Design review of the part built by this model. Coordinates are the model's own, in mm. A direction names the side the tool comes from. Coordinates: 2 decimals unless noted, no trailing zeros. Loops run counter-clockwise (first coordinate to the right, second up) from the corner with the lowest first, then second, coordinate; pieces in that order, holes last.
from build123d import *

# Parameters (mm, degrees)
BOSS_EXTRUDE1_DEPTH = 200
FILLET1_R           = 50
FILLET2_R           = 10
FILLET3_R           = 40
FILLET4_R           = 5
FILLET5_R           = 5
FILLET6_R           = 1
FILLET7_R           = 1
FILLET8_R           = 1
FILLET10_R          = 10
SHELL3_START        = 2
SHELL3_DEPTH        = 196
FILLET14_R          = 1
FILLET15_R          = 1
SKETCH5_W           = 165
SKETCH5_H           = 105
CUT_EXTRUDE1_DEPTH  = 20
SKETCH6_W           = 10
SKETCH6_H           = 3
CUT_EXTRUDE4_DEPTH  = 23
SKETCH8_R           = 7
CUT_EXTRUDE6_DEPTH  = 10
SKETCH9_R           = 10
SKETCH9_R_2         = 7.5
CUT_EXTRUDE7_DEPTH  = 3
SKETCH10_W          = 108
SKETCH10_H          = 2.810580917
SKETCH10_H_2        = 2.810580918
CUT_EXTRUDE8_DEPTH  = 3


# Read off the part's stored shape, not the designer's step: Shell3
with BuildPart() as part:
    # Sketch3 → Boss-Extrude1 (new body)
    with BuildSketch(Plane(origin=(0, 0, 0), x_dir=(0, 0, -1), z_dir=(1, 0, 0))):
        Polygon((-61.287916817, 93.76136528), (-140.28529736, -56.769076383), (39.71470264, -56.769076383), (39.71470264, -26.769076383), (0, -20.093366582), (0, 64.906633418), (22.555153974, 64.906633418), (22.555153974, 74.906633418), (4.646904738, 74.906633418), (4.646904738, 93.76136528), align=None)
    extrude(amount=BOSS_EXTRUDE1_DEPTH)

    # Fillet1
    fillet1_edges = [part.edges().sort_by_distance(p)[0] for p in [
        (100, 93.76136528, 61.287916817),
    ]]
    fillet(fillet1_edges, radius=FILLET1_R)

    # Fillet2
    fillet2_edges = [part.edges().sort_by_distance(p)[0] for p in [
        (100, -56.769076383, 140.28529736),
    ]]
    fillet(fillet2_edges, radius=FILLET2_R)

    # Fillet3
    fillet3_edges = [part.edges().sort_by_distance(p)[0] for p in [
        (100, -20.093366582, 0),
    ]]
    fillet(fillet3_edges, radius=FILLET3_R)

    # Fillet4
    fillet4_edges = [part.edges().sort_by_distance(p)[0] for p in [
        (100, -26.769076383, -39.71470264),
    ]]
    fillet(fillet4_edges, radius=FILLET4_R)

    # Fillet5
    fillet5_edges = [part.edges().sort_by_distance(p)[0] for p in [
        (100, 74.906633418, -4.646904738),
    ]]
    fillet(fillet5_edges, radius=FILLET5_R)

    # Fillet6
    fillet6_edges = [part.edges().sort_by_distance(p)[0] for p in [
        (100, 93.76136528, -4.646904738),
    ]]
    fillet(fillet6_edges, radius=FILLET6_R)

    # Fillet7
    fillet7_edges = [part.edges().sort_by_distance(p)[0] for p in [
        (100, 74.906633418, -22.555153974),
    ]]
    fillet(fillet7_edges, radius=FILLET7_R)

    # Fillet8
    fillet8_edges = [part.edges().sort_by_distance(p)[0] for p in [
        (100, 64.906633418, -22.555153974),
    ]]
    fillet(fillet8_edges, radius=FILLET8_R)

    # Fillet10
    fillet10_edges = [part.edges().sort_by_distance(p)[0] for p in [
        (100, 64.906633418, 0),
    ]]
    fillet(fillet10_edges, radius=FILLET10_R)

    # Shell3 outline → Shell3 (cut)
    with BuildSketch(Plane.YZ.offset(SHELL3_START)):
        with BuildLine():
            Line((-27.674806697, -33.037823142), (-25.702476507, -33.369355374))
            ThreePointArc((-25.702476507, -33.369355374), (-12.089709184, -9.461288624), (13.744127299, 0))
            Line((13.744127299, 0), (54.906633418, 0))
            Line((54.906633418, 0), (54.906633418, 2))
            ThreePointArc((54.906633418, 2), (63.391914792, -1.514718626), (66.906633418, -10))
            Line((66.906633418, -10), (66.906633418, -20.555153974))
            Line((66.906633418, -20.555153974), (72.906633418, -20.555153974))
            Line((72.906633418, -20.555153974), (72.906633418, -9.646904738))
            ThreePointArc((72.906633418, -9.646904738), (74.956885949, -4.697157269), (79.906633418, -2.646904738))
            Line((79.906633418, -2.646904738), (91.76136528, -2.646904738))
            Line((91.76136528, -2.646904738), (91.76136528, 31.060602511))
            ThreePointArc((91.76136528, 31.060602511), (84.838407844, 55.893576038), (66.066508022, 73.563315451))
            Line((66.066508022, 73.563315451), (-43.051552593, 130.82775222))
            ThreePointArc((-43.051552593, 130.82775222), (-50.907905305, 130.590140491), (-54.769076383, 123.74396673))
            Line((-54.769076383, 123.74396673), (-54.769076383, -37.71470264))
            Line((-54.769076383, -37.71470264), (-30.998763119, -37.71470264))
            ThreePointArc((-30.998763119, -37.71470264), (-29.061225382, -37.005105993), (-28.040267833, -35.212000987))
            Line((-28.040267833, -35.212000987), (-27.674806697, -33.037823142))
        make_face()
    extrude(amount=SHELL3_DEPTH, mode=Mode.SUBTRACT)

    # Fillet14
    fillet14_edges = [part.edges().sort_by_distance(p)[0] for p in [
        (200, -43.883919751, -39.71470264),
        (200, 12.436858662, 103.966480208),
        (200, 86.549951284, 56.928283268),
        (200, -56.769076383, 42.014632045),
        (200, -51.942612535, 132.301683931),
        (200, 34.325380359, 0),
        (200, -12.089709184, -9.461288624),
        (200, -25.885207075, -34.456444296),
        (200, -27.769533558, -38.532041562),
        (200, 86.333999349, -4.646904738),
        (200, 76.371099512, -6.111370832),
        (200, 93.76136528, 13.706848886),
        (200, 93.468472061, -4.354011519),
        (200, 74.906633418, -15.601029356),
        (200, 74.613740199, -22.262260756),
        (200, 69.906633418, -22.555153974),
        (200, 65.199526636, -22.262260756),
        (200, 64.906633418, -15.777576987),
        (200, 61.97770123, -2.928932188),
    ]]
    fillet(fillet14_edges, radius=FILLET14_R)

    # Fillet15
    fillet15_edges = [part.edges().sort_by_distance(p)[0] for p in [
        (0, -43.883919751, -39.71470264),
        (0, 12.436858662, 103.966480208),
        (0, 86.549951284, 56.928283268),
        (0, -56.769076383, 42.014632045),
        (0, -51.942612535, 132.301683931),
        (0, 34.325380359, 0),
        (0, -12.089709184, -9.461288624),
        (0, -25.885207075, -34.456444296),
        (0, -27.769533558, -38.532041562),
        (0, 86.333999349, -4.646904738),
        (0, 76.371099512, -6.111370832),
        (0, 93.76136528, 13.706848886),
        (0, 93.468472061, -4.354011519),
        (0, 74.906633418, -15.601029356),
        (0, 74.613740199, -22.262260756),
        (0, 69.906633418, -22.555153974),
        (0, 65.199526636, -22.262260756),
        (0, 64.906633418, -15.777576987),
        (0, 61.97770123, -2.928932188),
    ]]
    fillet(fillet15_edges, radius=FILLET15_R)

    # Sketch5 → Cut-Extrude1 (cut)
    with BuildSketch(Plane(origin=(0, 45.46476773, 86.633651895), x_dir=(1, 0, 0), z_dir=(0, 0.4646904737791423, 0.8854731862563182))):
        with Locations((100, -28.184050547)):
            Rectangle(SKETCH5_W, SKETCH5_H)
    extrude(amount=-CUT_EXTRUDE1_DEPTH, mode=Mode.SUBTRACT)

    # Sketch6 → Cut-Extrude4 (cut)
    with BuildSketch(Plane(origin=(0, 74.906633418, 0), x_dir=(1, 0, 0), z_dir=(0, 1, 0))):
        with Locations((179, 17.055153974)):
            Rectangle(SKETCH6_W, SKETCH6_H)
        with Locations((139, 17.055153974)):
            Rectangle(SKETCH6_W, SKETCH6_H)
        with Locations((99, 17.055153974)):
            Rectangle(SKETCH6_W, SKETCH6_H)
        with Locations((59, 17.055153974)):
            Rectangle(SKETCH6_W, SKETCH6_H)
        with Locations((19, 17.021146207)):
            Rectangle(SKETCH6_W, SKETCH6_H)
    extrude(amount=-CUT_EXTRUDE4_DEPTH, mode=Mode.SUBTRACT)

    # Sketch8 → Cut-Extrude6 (cut)
    with BuildSketch(Plane(origin=(0, 45.46476773, 86.633651895), x_dir=(1, 0, 0), z_dir=(0, 0.4646904737791423, 0.8854731862563182))):
        with Locations(Location((31, -90.684050547, 0), (0, 0, 270))):
            Circle(SKETCH8_R)
        with Locations(Location((169, -90.684050547, 0), (0, 0, 270))):
            Circle(SKETCH8_R)
    extrude(amount=-CUT_EXTRUDE6_DEPTH, mode=Mode.SUBTRACT)

    # Sketch9 → Cut-Extrude7 (cut)
    with BuildSketch(Plane(origin=(0, 0, -39.71470264), x_dir=(-1, 0, 0), z_dir=(0, 0, -1))):
        with Locations(Location((-179, -44.269076383, 0), (0, 0, 90))):
            Circle(SKETCH9_R)
        with Locations(Location((-149, -44.039846818, 0), (0, 0, 90))):
            Circle(SKETCH9_R)
        with Locations(Location((-119, -44.039846818, 0), (0, 0, 90))):
            Circle(SKETCH9_R)
        with Locations(Location((-89, -43.960489904, 0), (0, 0, 90))):
            Circle(SKETCH9_R)
        with Locations(Location((-59, -43.960489904, 0), (0, 0, 90))):
            Circle(SKETCH9_R)
        with Locations(Location((-21, -41.769076383, 0), (0, 0, 90))):
            Circle(SKETCH9_R_2)
    extrude(amount=-CUT_EXTRUDE7_DEPTH, mode=Mode.SUBTRACT)

    # Sketch10 → Cut-Extrude8 (cut)
    with BuildSketch(Plane(origin=(0, 45.46476773, 86.633651895), x_dir=(1, 0, 0), z_dir=(0, 0.46469047377914224, 0.8854731862563181))):
        with Locations((100, -87.49160573)):
            Rectangle(SKETCH10_W, SKETCH10_H)
        with Locations((100, -91.302186647)):
            Rectangle(SKETCH10_W, SKETCH10_H_2)
        with Locations((100, -95.112767565)):
            Rectangle(SKETCH10_W, SKETCH10_H_2)
    extrude(amount=-CUT_EXTRUDE8_DEPTH, mode=Mode.SUBTRACT)


solid = part.part
Q1. Take a section at B-B, the plane x = 59. Give the number of separate pieces and of enclosed holes in the cut face, then the cut area to 3 significant figures.
Q2. Take a section at A-A, the plane z = 15. Write out the cut boundary in (x, y), then the cut area to 3 significant figures.
Q3. Clearance check with flat-ended pins moving along their axes: pin 1 Ø1 at (x, y) = (60, 73.5) entering from +Z; pin 2 Ø9 at (x, y) = (95, 70.5) entering from -Z; pin 3 Ø0.5 at (x, y) = (198.5, 27.5) entering from -Z. State where each tip first meets the part, or that it passes through.
Q4. Machinability: for faces 1 (the cylindrical face through (101.39, 62.06, -3.01)), 2 (the flat face through (99, 91.761, 14)), 3 (the cylindrical face through (127.43, -38.66, -38.73)), which of the approach directions +Z, -Z, +X, -X, +Y, -Y give a long, thin tool a straight path to every point of the face, cutting with its end or side? Answer none if there is none.
Q5. The part is to be moulded in two halves that separate along Y. For faces 4 (the flat face through (106.87, -27.72, 125.04)), 5 (the cylindrical face through (37.94, -34.48, 127.48)), 6 (the flat face through (99, -47, -39.715)), 7 (the cylindrical face through (52.92, -51.9, -38.73)), say which applies: pulls with the +Y half, pulls with the -Y half, needs draft (parallel to the pull), parting line crosses it, or undercut.
Q6. For line 1 (Y direction, x = 117, z = -20); line 2 (Y direction, x = 86, z = 8); line 3 (X direction, y = 20.5, z = 18.5), list the stretches that pass through material, from the lowest coordinate up.
Entries:
1. separate pieces: 8
1. enclosed holes: 0
1. area: 712 mm2
2. outline: (0, -55.77) arc R1 ccw to (1, -56.77) - (199, -56.77) arc R1 ccw to (200, -55.77) - (200, 92.76) arc R1 ccw to (199, 93.76) - (1, 93.76) arc R1 ccw to (0, 92.76) - close; hole (2, -54.77) - (198, -54.77) - (198, 91.76) - (2, 91.76) - close
2. area: 1,390 mm2
3. pin 1: stops at z = 71.62
3. pin 2: stops at z = -22.56
3. pin 3: stops at z = 0
4. face 1: -Z, +X, -X
4. face 2: none
4. face 3: -Z
5. face 4: pulls with the +Y half
5. face 5: undercut
5. face 6: needs draft
5. face 7: undercut
6. line 1: y = -56.77 to -54.77, 64.91 to 66.91, 72.91 to 74.91
6. line 2: y = -56.77 to -54.77, 91.76 to 93.76
6. line 3: x = 0 to 2, 198 to 200
